Autodesk Inventor part; units mm, degrees
ref_plane "YZ Plane" through (0, 0, 0) normal (1, 0, 0) x (0, 1, 0)
ref_plane "XZ Plane" through (0, 0, 0) normal (0, 1, 0) x (-1, 0, 0)
ref_plane "XY Plane" through (0, 0, 0) normal (0, 0, 1) x (1, 0, 0)
sketch "Sketch1" plane through (0, 0, 0) normal (0, 1, 0) x (-1, 0, 0)
  line L0 (39.5855, 7.487) -> (-0.4145, 7.487)
  line L1 (-0.4145, 7.487) -> (-0.4145, -7.513)
  line L2 (-0.4145, -7.513) -> (39.5855, -7.513)
  line L3 (39.5855, -7.513) -> (39.5855, 7.487)
  point P0 (0, 0)
  dimension "d0" = 40
  dimension "d1" = 15
extrude "Extrusion1" add sketch "Sketch1" along normal blind 15
sketch "Sketch2" plane through (0, 15, 0) normal (0, 1, 0) x (1, 0, 0)
  line L0 (-39.5855, -7.487) -> (0.4145, -7.487)
  line L1 (-36.5855, -7.487) -> (-2.5855, -7.487)
  line L2 (-2.5855, -7.487) -> (-2.5855, 3.513)
  line L3 (-2.5855, 3.513) -> (-36.5855, 3.513)
  line L4 (-36.5855, 3.513) -> (-36.5855, -7.487)
  line L5 (0.4145, 7.513) -> (-39.5855, 7.513)
  line L6 (-39.5855, 7.513) -> (-39.5855, -7.487)
  line L7 (0.4145, -7.487) -> (0.4145, 7.513)
  point P0 (0, 0)
  dimension "d4" = 4
  dimension "d5" = 3
  dimension "d6" = 3
extrude "Extrusion2" cut sketch "Sketch2" against normal blind 11 contours L4 L3 L2 L0
sketch "Sketch3" plane through (-39.5855, 0, -7.513) normal (-1, 0, 0) x (0, 0, 1)
  circle A0 centre (10, 10) radius 1.4
  line L0 (15, 4) -> (4, 4)
  line L1 (4, 15) -> (4, 4)
  point P0 (7.513, 0)
  dimension "d9" = 2.8
  dimension "d10" = 6
  dimension "d11" = 6
extrude "Extrusion3" cut sketch "Sketch3" against normal through all
fillet "Fillet1" radius 1 1 edges at (-19.5855, 4, -3.513)
fillet "Fillet2" radius 1 3 edges at (-36.5855, 10, -3.513) (-36.5855, 4.2929, -3.2201) (-36.5855, 4, 2.487)
fillet "Fillet3" radius 1 3 edges at (-2.5855, 4, 2.487) (-2.5855, 4.2929, -3.2201) (-2.5855, 10, -3.513)
properties part number "leg_8"
Design review of the part built by this model. Coordinates are the model's own, in mm. A direction names the side the tool comes from. Give positions to 0.01 mm unless a question says otherwise; leave off trailing zeros. Loops run counter-clockwise (first coordinate to the right, second up) from the corner with the lowest first, then second, coordinate; pieces in that order, holes last. Notation, with made-up numbers: M -24.75,-32 L 18.25,-32 A21 cw 18.25,3 Z; hole C 9,-6.75 d6. An arc over 180 degrees is marked long. Return JSON: item names as keys, results as strings. Group by question number.
Item 1: Tool access review of faces 5 (the flat face through (-20, 2, 7.487)), 6 (the flat face through (-2.586, 9, 4)): name each direction out of +Z, -Z, +X, -X, +Y, -Y from which nothing blocks a thin tool from reaching the whole face with its end or side.
Item 2: Insertion check: pin 1 Ø8 at (y, z) = (11, 3) entering from -X; pin 2 Ø8 at (x, y) = (-23, 8.5) entering from +Z; pin 3 Ø3 at (x, z) = (-15.5, 4.5) entering from +Y; pin 4 Ø1 at (x, y) = (-31, 11) entering from +Z. Each pin has a flat end and moves straight along its axis. Give the tip position at first contact, or say it passes through.
Item 3: For probe 1 along X at (y, z) = (9.5, 6.5); probe 2 along Y at (x, z) = (-31, 1.5); probe 3 along X at (y, z) = (4.5, 5.5), list the stretches that pass through material, from the lowest coordinate up.
Item 4: We need section B-B (x = -17.5). Give the boundary of the cut face in (y, z), and give its area (3 significant figures).
Item 5: We need section D-D (y = 5.75). Give the boundary of the cut face in (x, z).
Item 6: Mouldability with a two-part tool opening along X and no side actions: class faces 1 (the cylindrical face through (-36.3, 4.3, 2.6)), 2 (the flat face through (0.414, 7, 0)), 3 (the cylindrical face through (-1.11, 10.95, 1.46)), 4 (the cylindrical face through (-36.3, 9.93, -3.21)) as released by +X, released by -X, zero draft, split by the parting line, or undercut.
Item 7: We need section A-A (y = 10). Give the boundary of the cut face in (x, z).
Item 8: We need section C-C (z = 3). Give the boundary of the cut face in (x, y).
Output:
{
 "1": {"face 5": "+Z, +X, -X, +Y, -Y", "face 6": "+Z, +Y"},
 "2": {"pin 1": "stops at x = -39.59", "pin 2": "stops at z = -3.38", "pin 3": "stops at y = 4", "pin 4": "stops at z = -3.51"},
 "3": {"probe 1": "x = -39.59 to -36.59, -2.59 to 0.41", "probe 2": "y = 0 to 4", "probe 3": "x = -39.59 to -36.45, -2.72 to 0.41"},
 "4": {"outline": "M 0,-7.51 L 15,-7.51 L 15,-3.51 L 5,-3.51 A1 cw 4,-2.51 L 4,7.49 L 0,7.49 Z", "area": "104 mm^2"},
 "5": {"outline": "M -39.59,-7.51 L 0.41,-7.51 L 0.41,7.49 L -2.59,7.49 L -2.59,-2.51 A1 cw -3.59,-3.51 L -35.59,-3.51 A1 cw -36.59,-2.51 L -36.59,7.49 L -39.59,7.49 Z"},
 "6": {"face 1": "undercut", "face 2": "released by +X", "face 3": "zero draft", "face 4": "undercut"},
 "7": {"outline": "M -39.59,-7.51 L 0.41,-7.51 L 0.41,1.09 L -2.59,1.09 L -2.59,-2.51 A1 cw -3.59,-3.51 L -35.59,-3.51 A1 cw -36.59,-2.51 L -36.59,1.09 L -39.59,1.09 Z; M -39.59,3.89 L -36.59,3.89 L -36.59,7.49 L -39.59,7.49 Z; M -2.59,3.89 L 0.41,3.89 L 0.41,7.49 L -2.59,7.49 Z"},
 "8": {"outline": "M -39.59,0 L 0.41,0 L 0.41,8.7 L -2.59,8.7 L -2.59,5 A1 cw -3.59,4 L -35.59,4 A1 cw -36.59,5 L -36.59,8.7 L -39.59,8.7 Z; M -39.59,11.3 L -36.59,11.3 L -36.59,15 L -39.59,15 Z; M -2.59,11.3 L 0.41,11.3 L 0.41,15 L -2.59,15 Z"}
}
